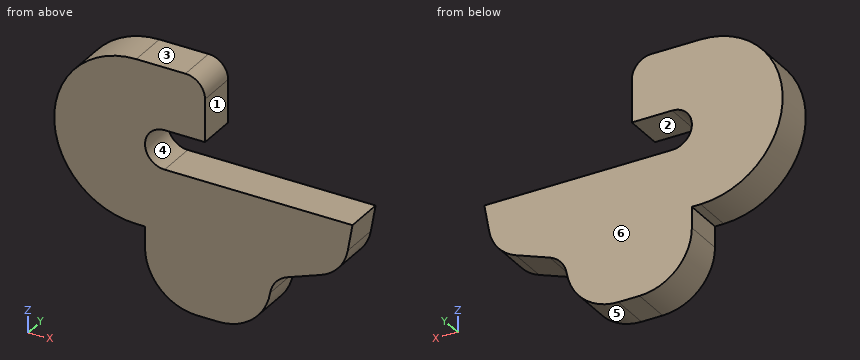
```python
from build123d import *

# Parameters (mm, degrees)
BOSS_EXTRUDE2_DEPTH = 3


with BuildPart() as part:
    # Sketch1 → Boss-Extrude2 (new body)
    with BuildSketch(Plane(origin=(0, 0, 0), x_dir=(1, 0, 0), z_dir=(0, 1, 0))):
        with BuildLine():
            Line((0, 0), (-3.09, 0))
            ThreePointArc((-3.09, 0), (-4.59, 1.5), (-3.09, 3))
            Line((-3.09, 3), (11.27, 3))
            Line((11.27, 3), (10.908822115, 5.04834157))
            ThreePointArc((10.908822115, 5.04834157), (10.208482238, 6.549941992), (8.851032589, 7.5))
            Line((8.851032589, 7.5), (6.27, 8.438574292))
            ThreePointArc((6.27, 8.438574292), (5.411457646, 9.044534587), (4.978627211, 10.002104777))
            ThreePointArc((4.978627211, 10.002104777), (3.62422767, 12.413716405), (1.02888753, 13.37))
            Line((1.02888753, 13.37), (-0.59, 13.37))
            ThreePointArc((-0.59, 13.37), (-3.418427125, 12.198427125), (-4.59, 9.37))
            Line((-4.59, 9.37), (-4.59, 7.77))
            Line((-4.59, 7.77), (-5.26, 7.77))
            ThreePointArc((-5.26, 7.77), (-11.53, 1.5), (-5.26, -4.77))
            Line((-5.26, -4.77), (-1.5, -4.77))
            ThreePointArc((-1.5, -4.77), (-0.439339828, -4.330660172), (0, -3.27))
            Line((0, -3.27), (0, 0))
        make_face()
    extrude(amount=BOSS_EXTRUDE2_DEPTH)


solid = part.part
```
CAD build for the part. Positions are in the model's coordinates, mm. Face numbers are marked on the shaded views. A direction names the side the tool comes from. Round coordinates to 2 decimals unless told otherwise and drop trailing zeros. Order: outer loops, then holes, each group sorted by start corner. A loop starts at its lowest first (then second) coordinate and runs counter-clockwise, first axis right, second up.
Item 1: Mould opens along Z. For the marked faces 4, 5 and 6 say: pulls with the +Z half, pulls with the -Z half, needs draft (parallel to the pull), parting line crosses it, or undercut.
Item 2: Probe line 1 along Z through (x, y) = (-3, 1.5); line 2 along Z through (x, y) = (-1, 0.65); line 3 along X through (y, z) = (0.8, -5). List the from-to ranges inside material, lowest first.
Item 3: Tool access for the marked faces 1, 2 and 3: list every direction of +Z, -Z, +X, -X, +Y, -Y with a clear straight run to the whole face (end or side of a thin tool).
Item 4: Saw through at A-A on x = -1. Write the cut outline in (y, z).
Item 5: Pin check, flat tips, straight feed: pin 1 (1 mm diameter, centred on x = 3.5, y = 1, fed in from -Z); pin 2 (1.5 mm diameter, centred on x = -2, y = 1, fed in from -Z). Stop position of each tip, or through.
Item 6: Saw through at C-C on z = -1.5. Write the cut outline in (x, y).
Item 7: Saw through at B-B on y = 1.1. Write the cut outline in (x, z), then the cut area to 3 significant figures.
Item 8: Saw through at D-D on x = -8.75. Write the cut outline in (y, z).
Reported:
1. face 4: undercut
1. face 5: pulls with the -Z half
1. face 6: needs draft
2. line 1: z = -12.56 to -3, 0 to 4.77
2. line 2: z = -13.35 to -3, 0 to 4.68
2. line 3: x = -10.46 to 10.92
3. face 1: +Z, +X, +Y, -Y
3. face 2: +X, +Y, -Y
3. face 3: +Z, +X, -X, +Y, -Y
4. outline: (0, -13.35) - (3, -13.35) - (3, -3) - (0, -3) - close; (0, 0) - (3, 0) - (3, 4.68) - (0, 4.68) - close
5. pin 1: stops at z = -12.85
5. pin 2: stops at z = -13.32
6. outline: (-11.53, 0) - (-4.59, 0) - (-4.59, 3) - (-11.53, 3) - close
7. outline: (-5.26, -7.77) - (-4.59, -7.77) - (-4.59, -9.37) arc R4 ccw to (-0.59, -13.37) - (1.03, -13.37) arc R4 ccw to (4.98, -10) arc R2 cw to (6.27, -8.44) - (8.85, -7.5) arc R3.2 ccw to (10.91, -5.05) - (11.27, -3) - (-3.09, -3) arc R1.5 cw to (-3.09, 0) - (0, 0) - (0, 3.27) arc R1.5 ccw to (-1.5, 4.77) - (-5.26, 4.77) arc R6.27 ccw to start
7. area: 214 mm2
8. outline: (0, -6.71) - (3, -6.71) - (3, 3.71) - (0, 3.71) - close
